Here's how the part is built. I have some questions about the finished solid (model axes, mm). Give positions to 0.01 mm unless a question says otherwise; leave off trailing zeros. Write each loop counter-clockwise with the first axis right and the second up, starting at its lowest first coordinate (ties: lowest second). Pieces come first, ordered by that corner, then holes. Notation, with made-up numbers: (31.5, 75.5) - (49.5, 75.5) arc R25 ccw to (49.5, 104.5) - close; hole circle Ø4 at (8.5, -31). An arc over 180 degrees is marked (long way). Write each question's results on one line, items separated by ' | '. Start each with the question number.
Item 1: Suppose I cut it at D-D on y = 77. List the corners of the cut face in (x, z) for me, then the cut area to 3 significant figures.
Item 2: Suppose I cut it at C-C on z = 0.25. List the corners of the cut face in (x, y) for me.
Item 3: Please list where these lines run through material, in increasing order: line 1 along X through (y, z) = (43, 0.5); line 2 along Y through (x, z) = (-25.5, -1.5); line 3 along Z through (x, y) = (-31, 4).
Item 4: Suppose I cut it at B-B on x = -1.5. List the corners of the cut face in (y, z) for me, then the cut area to 3 significant figures.
Item 5: Will these pins go through, and if not, where does the flat tip stop? P1, Ø4, axis at x = -21.5, z = -8.5, coming from the -Y side; P2, Ø2.5, axis at y = 92, z = 1.5, coming from the +X side; P3, Ø0.6, axis at y = 91.5, z = -2, coming from the +X side; P4, Ø12, axis at y = 13.5, z = 7.5, coming from the -X side.
Item 6: Suppose I cut it at A-A on y = 88.5. List the corners of the cut face in (x, z) for me.
```python
from build123d import *

# Parameters (mm, degrees)
BOSS_EXTRUDE1_DEPTH = 97
SKETCH2_W           = 12
SKETCH2_H           = 4.72
CUT_EXTRUDE1_DEPTH  = 10


with BuildPart() as part:
    # Sketch1 → Boss-Extrude1 (new body)
    with BuildSketch(Plane(origin=(0, 0, 0), x_dir=(1, 0, 0), z_dir=(0, 1, 0))):
        with BuildLine():
            Line((-28.95, 11.05), (28.95, 11.05))
            ThreePointArc((28.95, 11.05), (40, 0), (28.95, -11.05))
            Line((28.95, -11.05), (-28.95, -11.05))
            ThreePointArc((-28.95, -11.05), (-40, 0), (-28.95, 11.05))
        make_face()
    extrude(amount=BOSS_EXTRUDE1_DEPTH)

    # Sketch2 → Cut-Extrude1 (cut)
    with BuildSketch(Plane(origin=(0, 97, 0), x_dir=(1, 0, 0), z_dir=(0, 1, 0))):
        with Locations((-25, -0.69)):
            Rectangle(SKETCH2_W, SKETCH2_H)
        with Locations((-5.4, -0.69)):
            Rectangle(SKETCH2_W, SKETCH2_H)
        Polygon((25.45, 0.8), (24.45, 1.8), (24.45, 3.05), (31.75, 3.05), (31.75, 1.8), (30.75, 0.8), align=None)
    extrude(amount=-CUT_EXTRUDE1_DEPTH, mode=Mode.SUBTRACT)


solid = part.part
```
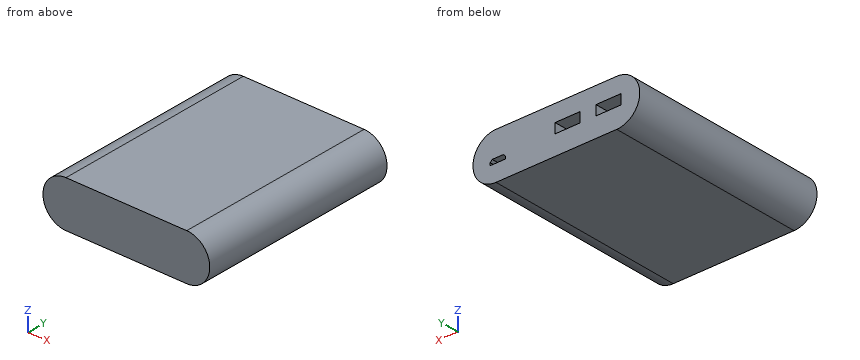
Checked values:
1) outline: (-28.95, -11.05) - (28.95, -11.05) arc R11.05 ccw to (28.95, 11.05) - (-28.95, 11.05) arc R11.05 ccw to start | area: 1,660 mm^2
2) outline: (-40, 0) - (40, 0) - (40, 97) - (0.6, 97) - (0.6, 87) - (-11.4, 87) - (-11.4, 97) - (-19, 97) - (-19, 87) - (-31, 87) - (-31, 97) - (-40, 97) - close
3) line 1: x = -39.99 to 39.99 | line 2: y = 0 to 87 | line 3: z = -10.86 to 10.86
4) outline: (0, -11.05) - (97, -11.05) - (97, -1.67) - (87, -1.67) - (87, 3.05) - (97, 3.05) - (97, 11.05) - (0, 11.05) - close | area: 2,100 mm^2
5) P1: stops at y = 0 | P2: stops at x = 40 | P3: stops at x = 39.87 | P4: stops at x = -39.9
6) outline: (-28.95, -11.05) - (28.95, -11.05) arc R11.05 ccw to (28.95, 11.05) - (-28.95, 11.05) arc R11.05 ccw to start; hole (-31, -1.67) - (-19, -1.67) - (-19, 3.05) - (-31, 3.05) - close; hole (-11.4, -1.67) - (0.6, -1.67) - (0.6, 3.05) - (-11.4, 3.05) - close; hole (24.45, -3.05) - (31.75, -3.05) - (31.75, -1.8) - (30.75, -0.8) - (25.45, -0.8) - (24.45, -1.8) - close
